Read the model definition and answer for the solid it produces. Units are mm, in the model's axes. Face numbers are marked on the shaded views. A direction names the side the tool comes from. Give positions to 0.01 mm unless a question says otherwise; leave off trailing zeros. Write each loop counter-clockwise with the first axis right and the second up, starting at its lowest first coordinate (ties: lowest second). Pieces come first, ordered by that corner, then holes. Notation, with made-up numbers: M -26,70 L -12,70 A19 cw -12,97 Z; hole C -11.5,28 d8. An arc over 180 degrees is marked long. Use a Markdown table: item, result. Add a question column.
Item 1: A cutting plane is placed at B-B on y = 12.25. Determine the outline of the cut face in (x, z), then the cut area to 3 significant figures.
Item 2: A cutting plane is placed at C-C on y = 21.25. Determine the outline of the cut face in (x, z).
Item 3: A cutting plane is placed at A-A on x = 35.25. Determine the outline of the cut face in (y, z), then the cut area to 3 significant figures.
Item 4: Given P1, Ø10, axis at y = 10.5, z = 39.5, coming from the -X side; P2, Ø5.5, axis at y = 15.5, z = 17, coming from the +X side; P3, Ø6, axis at y = 11.5, z = 41, coming from the +X side; P4, Ø2, axis at x = 36.5, z = 46, coming from the +Y side, each flat-ended and moving along its own axis, determine where each tip first touches the part or whether it passes through.
Item 5: Consider probe 1 along Y at (x, z) = (33.25, 22); probe 2 along Z at (x, y) = (38.25, 15); probe 3 along Y at (x, z) = (37.75, 50). Determine where each line is inside the solid, lowest interval first. Write a range as [from, to].
Item 6: A cutting plane is placed at D-D on z = 16. Determine the outline of the cut face in (x, y), then the cut area to 3 significant figures.
Item 7: For the marked faces 1, 2 and 3, determine the directions among +Z, -Z, +X, -X, +Y, -Y from which every point of the face is accessible in a straight line to the end or side of a thin tool.
from build123d import *

# Parameters (mm, degrees)
EXTRUDE025_DEPTH                          = 4
EXTRUDE024_DEPTH                          = 4
EXTRUDE024_ONTO_SKETCH023_PLACEMENT_ANGLE = 120


with BuildPart() as extrude025:
    # Sketch024 (on Face7 of Extrude024) → Extrude025 (new body)
    with BuildSketch(Plane(origin=(32.5, 0, 0), x_dir=(0, -1, 0), z_dir=(-1, 0, 0))):
        Polygon((-19, 10), (-22.458142, 20.240827), (-16.99404, 21.704929), (-11, 10), align=None)
    extrude(amount=-EXTRUDE025_DEPTH)


with BuildPart() as pin_reset:
    # Sketch023 as drawn → Extrude024 (new)
    with BuildSketch(Plane.XY):
        Polygon((32.5, 10.3), (36.5, 10.3), (36.5, 44.3), (40.5, 44.3), (40.5, 6.3), (36.5, 6.3), (32.5, 6.3), align=None)
    extrude(amount=EXTRUDE024_DEPTH)


with BuildPart() as pin_reset_1:
    # Extrude024 onto Sketch023 placement: moved
    add(pin_reset.part.moved(Location((0, 25.608142, 14.784867))).rotate(Axis((0, 25.608142, 14.784867), (1, 0, 0)), EXTRUDE024_ONTO_SKETCH023_PLACEMENT_ANGLE))

    # Connect006: union Extrude025
    add(extrude025.part)


solid = pin_reset_1.part
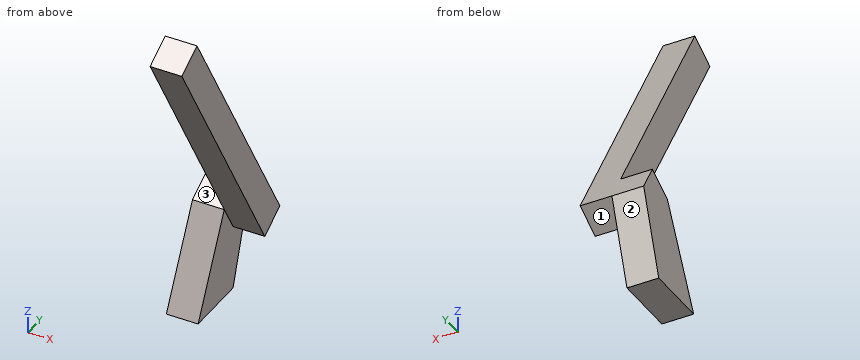
Filled in:
| question | item | result |
|---|---|---|
| 1 | outline | M 32.5,10 L 36.5,10 L 36.5,12.44 L 32.5,12.44 Z; M 36.5,29.92 L 40.5,29.92 L 40.5,37.92 L 36.5,37.92 Z |
| 1 | area | 41.8 mm² |
| 2 | outline | M 32.5,16.66 L 36.5,16.66 L 36.5,19.54 L 40.5,19.54 L 40.5,22.33 L 32.5,22.33 Z |
| 3 | outline | M 11,10 L 19,10 L 22.46,20.24 L 20.46,23.7 L 16.99,21.7 Z |
| 3 | area | 85.3 mm² |
| 4 | P1 | x = 36.5 |
| 4 | P2 | x = 36.5 |
| 4 | P3 | x = 40.5 |
| 4 | P4 | y = 8.16 |
| 5 | probe 1 | [17.51, 21.44] |
| 5 | probe 2 | [25.16, 33.16] |
| 5 | probe 3 | [0.66, 5.28] |
| 6 | outline | M 32.5,14.07 L 36.5,14.07 L 36.5,21.03 L 32.5,21.03 Z |
| 6 | area | 27.8 mm² |
| 7 | face 1 | -Z, +X, +Y |
| 7 | face 2 | -Z, +X, -X, +Y |
| 7 | face 3 | +Z, -X, -Y |
